Geometry: final body of the model. Coordinates: model frame, mm. A direction names the side the tool comes from. Give positions to 0.01 mm unless a question says otherwise; leave off trailing zeros. Write each loop counter-clockwise with the first axis right and the second up, starting at its lowest first coordinate (ties: lowest second). Pieces come first, ordered by that corner, then holes. Notation, with made-up numbers: (79.5, -28.5) -> (111.5, -28.5) arc R16 ccw to (111.5, -22.5) -> close; hole circle Ø7 at (75.25, -4). An arc over 180 degrees is marked (long way). Answer as a JSON object with one key per item and string values.
from build123d import *

# Parameters (mm, degrees)
SKETCH1_W               = 100
SKETCH1_H               = 100
BOSS_EXTRUDE1_DEPTH     = 100
SKETCH2_R               = 20
CUT_EXTRUDE1_DEPTH      = 5
CUT_EXTRUDE2_START      = -5
SKETCH3_R               = 20
CUT_EXTRUDE2_DEPTH      = 5
CUT_EXTRUDE3_DEPTH      = 151
CUT_EXTRUDE5_DEPTH      = 151
CUT_EXTRUDE5_DEPTH_BACK = 151
CUT_EXTRUDE6_DEPTH      = 151
CUT_EXTRUDE6_DEPTH_BACK = 151
FILLET3_R               = 2.5
BOSS_EXTRUDE3_DEPTH     = 10
CUT_EXTRUDE8_DEPTH      = 10
CUT_EXTRUDE9_DEPTH      = 10
BOSS_EXTRUDE4_DEPTH     = 10
CUT_EXTRUDE11_DEPTH     = 10
CUT_EXTRUDE12_DEPTH     = 10
BOSS_EXTRUDE5_DEPTH     = 10
CUT_EXTRUDE13_DEPTH     = 10
CUT_EXTRUDE15_DEPTH     = 10
BOSS_EXTRUDE6_DEPTH     = 10
CUT_EXTRUDE16_DEPTH     = 10
CUT_EXTRUDE17_DEPTH     = 10
BOSS_EXTRUDE7_DEPTH     = 10
CUT_EXTRUDE18_DEPTH     = 10
CUT_EXTRUDE19_DEPTH     = 10
BOSS_EXTRUDE8_DEPTH     = 10
CUT_EXTRUDE20_DEPTH     = 10
CUT_EXTRUDE21_DEPTH     = 10
BOSS_EXTRUDE9_DEPTH     = 10
CUT_EXTRUDE22_DEPTH     = 10
CUT_EXTRUDE23_DEPTH     = 10
BOSS_EXTRUDE10_DEPTH    = 10
CUT_EXTRUDE24_DEPTH     = 10
CUT_EXTRUDE25_DEPTH     = 10


with BuildPart() as part:
    # Sketch1 → Boss-Extrude1 (new body)
    with BuildSketch(Plane(origin=(0, 0, 0), x_dir=(0, 0, -1), z_dir=(1, 0, 0))):
        Rectangle(SKETCH1_W, SKETCH1_H)
    extrude(amount=BOSS_EXTRUDE1_DEPTH)

    # Sketch2 → Cut-Extrude1 (cut)
    with BuildSketch(Plane.ZY):
        Circle(SKETCH2_R)
    extrude(amount=-CUT_EXTRUDE1_DEPTH, mode=Mode.SUBTRACT)

    # Sketch3 → Cut-Extrude2 (cut)
    with BuildSketch(Plane(origin=(100, 0, 0), x_dir=(0, 0, -1), z_dir=(1, 0, 0)).offset(CUT_EXTRUDE2_START)):
        with Locations(Location((0, 0, 0), (0, 0, 180))):
            Circle(SKETCH3_R)
    extrude(amount=CUT_EXTRUDE2_DEPTH, mode=Mode.SUBTRACT)

    # Sketch4 → Cut-Extrude3 (cut, through all)
    with BuildSketch(Plane(origin=(0, 0, -50), x_dir=(-1, 0, 0), z_dir=(0, 0, -1))):
        Polygon((-80.128941466, 34.659382406), (-18.986632905, 34.659382406), (-9.691227462, 0), (-18.986632905, -35.340617594), (-80.128941466, -35.340617594), (-89.691227462, 0), align=None)
    extrude(amount=-CUT_EXTRUDE3_DEPTH, mode=Mode.SUBTRACT)

    # Sketch15 → Cut-Extrude5 (cut, two sides: drawn at the far end of the back side and taken through both)
    with BuildSketch(Plane(origin=(0, 50, 0), x_dir=(1, 0, 0), z_dir=(0, 1, 0)).offset(-CUT_EXTRUDE5_DEPTH_BACK)):
        with BuildLine():
            Line((75, -310), (75, -50))
            ThreePointArc((75, -50), (50, -25), (25, -50))
            Line((25, -50), (25, -310))
            Line((25, -310), (25, -830))
            Line((25, -830), (75, -830))
            Line((75, -830), (75, -310))
        make_face()
    extrude(amount=CUT_EXTRUDE5_DEPTH + CUT_EXTRUDE5_DEPTH_BACK, mode=Mode.SUBTRACT)

    # Sketch16 → Cut-Extrude6 (cut, two sides: drawn at the far end of the back side and taken through both)
    with BuildSketch(Plane(origin=(0, 50, 0), x_dir=(1, 0, 0), z_dir=(0, 1, 0)).offset(-CUT_EXTRUDE6_DEPTH_BACK)):
        with BuildLine():
            Line((25, 310), (25, 50))
            ThreePointArc((25, 50), (50, 25), (75, 50))
            Line((75, 50), (75, 310))
            Line((75, 310), (75, 830))
            Line((75, 830), (25, 830))
            Line((25, 830), (25, 310))
        make_face()
    extrude(amount=CUT_EXTRUDE6_DEPTH + CUT_EXTRUDE6_DEPTH_BACK, mode=Mode.SUBTRACT)

    # Fillet3
    fillet3_edges = [part.edges().sort_by_distance(p)[0] for p in [
        (50, -50, 25),
        (50, 50, 25),
        (50, -50, -25),
        (50, 50, -25),
    ]]
    fillet(fillet3_edges, radius=FILLET3_R)

    # Sketch17 → Boss-Extrude3 (add)
    with BuildSketch(Plane.XY.offset(50)):
        with BuildLine():
            Line((84.621199284, 43.079691203), (92.621199284, 43.079691203))
            ThreePointArc((92.621199284, 43.079691203), (94.621199284, 41.079691203), (92.621199284, 39.079691203))
            Line((92.621199284, 39.079691203), (84.621199284, 39.079691203))
            ThreePointArc((84.621199284, 39.079691203), (82.621199284, 41.079691203), (84.621199284, 43.079691203))
        make_face()
    extrude(amount=BOSS_EXTRUDE3_DEPTH)

    # Sketch18 → Cut-Extrude8 (cut)
    with BuildSketch(Plane(origin=(0, 43.079691203, 0), x_dir=(1, 0, 0), z_dir=(0, 1, 0))):
        Polygon((84.621199284, -50), (86.121199284, -60), (82.621199284, -60), (82.621199284, -50), align=None)
    extrude(amount=-CUT_EXTRUDE8_DEPTH, mode=Mode.SUBTRACT)

    # Sketch20 → Cut-Extrude9 (cut)
    with BuildSketch(Plane(origin=(0, 43.079691203, 0), x_dir=(1, 0, 0), z_dir=(0, 1, 0))):
        Polygon((91.121199284, -60), (94.621199284, -60), (94.621199284, -50), (92.621199284, -50), align=None)
    extrude(amount=-CUT_EXTRUDE9_DEPTH, mode=Mode.SUBTRACT)

    # Sketch24 → Boss-Extrude4 (add)
    with BuildSketch(Plane.XY.offset(50)):
        with BuildLine():
            Line((5.882221412, 43.579691203), (13.882221412, 43.579691203))
            ThreePointArc((13.882221412, 43.579691203), (16.382221412, 41.079691203), (13.882221412, 38.579691203))
            Line((13.882221412, 38.579691203), (5.882221412, 38.579691203))
            ThreePointArc((5.882221412, 38.579691203), (3.382221412, 41.079691203), (5.882221412, 43.579691203))
        make_face()
    extrude(amount=BOSS_EXTRUDE4_DEPTH)

    # Sketch25 → Cut-Extrude11 (cut)
    with BuildSketch(Plane(origin=(0, 43.579691203, 0), x_dir=(1, 0, 0), z_dir=(0, 1, 0))):
        Polygon((3.382221412, -50), (5.882221412, -50), (7.382221412, -60), (3.382221412, -60), align=None)
    extrude(amount=-CUT_EXTRUDE11_DEPTH, mode=Mode.SUBTRACT)

    # Sketch26 → Cut-Extrude12 (cut)
    with BuildSketch(Plane(origin=(0, 43.579691203, 0), x_dir=(1, 0, 0), z_dir=(0, 1, 0))):
        Polygon((12.382221412, -60), (13.882221412, -50), (16.382221412, -50), (16.382221412, -60), align=None)
    extrude(amount=-CUT_EXTRUDE12_DEPTH, mode=Mode.SUBTRACT)

    # Sketch27 → Boss-Extrude5 (add)
    with BuildSketch(Plane.XY.offset(50)):
        with BuildLine():
            Line((6.7978639, -43.920308797), (14.7978639, -43.920308797))
            ThreePointArc((14.7978639, -43.920308797), (17.2978639, -41.420308797), (14.7978639, -38.920308797))
            Line((14.7978639, -38.920308797), (6.7978639, -38.920308797))
            ThreePointArc((6.7978639, -38.920308797), (4.2978639, -41.420308797), (6.7978639, -43.920308797))
        make_face()
    extrude(amount=BOSS_EXTRUDE5_DEPTH)

    # Sketch29 → Cut-Extrude13 (cut)
    with BuildSketch(Plane.XZ.offset(43.920308797)):
        Polygon((8.2978639, 60), (6.7978639, 50), (4.2978639, 50), (4.2978639, 60), align=None)
    extrude(amount=-CUT_EXTRUDE13_DEPTH, mode=Mode.SUBTRACT)

    # Sketch30 → Cut-Extrude15 (cut)
    with BuildSketch(Plane.XZ.offset(43.920308797)):
        Polygon((14.0478639, 60), (17.2978639, 60), (17.2978639, 50), (14.7978639, 50), align=None)
    extrude(amount=-CUT_EXTRUDE15_DEPTH, mode=Mode.SUBTRACT)

    # Sketch31 → Boss-Extrude6 (add)
    with BuildSketch(Plane.XY.offset(50)):
        with BuildLine():
            Line((82.517325635, -38.920308797), (90.517325635, -38.920308797))
            ThreePointArc((90.517325635, -38.920308797), (93.017325635, -41.420308797), (90.517325635, -43.920308797))
            Line((90.517325635, -43.920308797), (82.517325635, -43.920308797))
            ThreePointArc((82.517325635, -43.920308797), (80.017325635, -41.420308797), (82.517325635, -38.920308797))
        make_face()
    extrude(amount=BOSS_EXTRUDE6_DEPTH)

    # Sketch33 → Cut-Extrude16 (cut)
    with BuildSketch(Plane.XZ.offset(43.920308797)):
        Polygon((83.621199284, 60), (82.517325635, 50), (80.017325635, 50), (80.017325635, 60), align=None)
    extrude(amount=-CUT_EXTRUDE16_DEPTH, mode=Mode.SUBTRACT)

    # Sketch34 → Cut-Extrude17 (cut)
    with BuildSketch(Plane.XZ.offset(43.920308797)):
        Polygon((89.56926246, 60), (90.517325635, 50), (93.017325635, 50), (93.017325635, 60), align=None)
    extrude(amount=-CUT_EXTRUDE17_DEPTH, mode=Mode.SUBTRACT)

    # Sketch35 → Boss-Extrude7 (add)
    with BuildSketch(Plane(origin=(0, 0, -50), x_dir=(-1, 0, 0), z_dir=(0, 0, -1))):
        with BuildLine():
            Line((-17.608468635, 43.579691203), (-9.608468635, 43.579691203))
            ThreePointArc((-9.608468635, 43.579691203), (-7.108468635, 41.079691203), (-9.608468635, 38.579691203))
            Line((-9.608468635, 38.579691203), (-17.608468635, 38.579691203))
            ThreePointArc((-17.608468635, 38.579691203), (-20.108468635, 41.079691203), (-17.608468635, 43.579691203))
        make_face()
    extrude(amount=BOSS_EXTRUDE7_DEPTH)

    # Sketch36 → Cut-Extrude18 (cut)
    with BuildSketch(Plane(origin=(0, 43.579691203, 0), x_dir=(1, 0, 0), z_dir=(0, 1, 0))):
        Polygon((11.108468635, 60), (9.608468635, 50), (7.108468635, 50), (7.108468635, 60), align=None)
    extrude(amount=-CUT_EXTRUDE18_DEPTH, mode=Mode.SUBTRACT)

    # Sketch37 → Cut-Extrude19 (cut)
    with BuildSketch(Plane(origin=(0, 43.579691203, 0), x_dir=(1, 0, 0), z_dir=(0, 1, 0))):
        Polygon((16.858468635, 60), (17.608468635, 50), (20.108468635, 50), (20.108468635, 60), align=None)
    extrude(amount=-CUT_EXTRUDE19_DEPTH, mode=Mode.SUBTRACT)

    # Sketch38 → Boss-Extrude8 (add)
    with BuildSketch(Plane(origin=(0, 0, -50), x_dir=(-1, 0, 0), z_dir=(0, 0, -1))):
        with BuildLine():
            Line((-17.330505729, -38.920308797), (-9.330505729, -38.920308797))
            ThreePointArc((-9.330505729, -38.920308797), (-6.830505729, -41.420308797), (-9.330505729, -43.920308797))
            Line((-9.330505729, -43.920308797), (-17.330505729, -43.920308797))
            ThreePointArc((-17.330505729, -43.920308797), (-19.830505729, -41.420308797), (-17.330505729, -38.920308797))
        make_face()
    extrude(amount=BOSS_EXTRUDE8_DEPTH)

    # Sketch40 → Cut-Extrude20 (cut)
    with BuildSketch(Plane.XZ.offset(43.920308797)):
        Polygon((10.830505729, -60), (9.330505729, -50), (6.830505729, -50), (6.830505729, -60), align=None)
    extrude(amount=-CUT_EXTRUDE20_DEPTH, mode=Mode.SUBTRACT)

    # Sketch41 → Cut-Extrude21 (cut)
    with BuildSketch(Plane.XZ.offset(43.920308797)):
        Polygon((16.580505729, -60), (17.330505729, -50), (19.830505729, -50), (19.830505729, -60), align=None)
    extrude(amount=-CUT_EXTRUDE21_DEPTH, mode=Mode.SUBTRACT)

    # Sketch42 → Boss-Extrude9 (add)
    with BuildSketch(Plane(origin=(0, 0, -50), x_dir=(-1, 0, 0), z_dir=(0, 0, -1))):
        with BuildLine():
            Line((-94.397005035, 43.579691203), (-86.397005035, 43.579691203))
            ThreePointArc((-86.397005035, 43.579691203), (-83.897005035, 41.079691203), (-86.397005035, 38.579691203))
            Line((-86.397005035, 38.579691203), (-94.397005035, 38.579691203))
            ThreePointArc((-94.397005035, 38.579691203), (-96.897005035, 41.079691203), (-94.397005035, 43.579691203))
        make_face()
    extrude(amount=BOSS_EXTRUDE9_DEPTH)

    # Sketch43 → Cut-Extrude22 (cut)
    with BuildSketch(Plane(origin=(0, 43.579691203, 0), x_dir=(1, 0, 0), z_dir=(0, 1, 0))):
        Polygon((87.897005035, 60), (86.397005035, 50), (83.897005035, 50), (83.897005035, 60), align=None)
    extrude(amount=-CUT_EXTRUDE22_DEPTH, mode=Mode.SUBTRACT)

    # Sketch44 → Cut-Extrude23 (cut)
    with BuildSketch(Plane(origin=(0, 43.579691203, 0), x_dir=(1, 0, 0), z_dir=(0, 1, 0))):
        Polygon((93.647005035, 60), (94.397005035, 50), (96.897005035, 50), (96.897005035, 60), align=None)
    extrude(amount=-CUT_EXTRUDE23_DEPTH, mode=Mode.SUBTRACT)

    # Sketch45 → Boss-Extrude10 (add)
    with BuildSketch(Plane(origin=(0, 0, -50), x_dir=(-1, 0, 0), z_dir=(0, 0, -1))):
        with BuildLine():
            Line((-93.140486024, -38.920308797), (-85.140486024, -38.920308797))
            ThreePointArc((-85.140486024, -38.920308797), (-82.640486024, -41.420308797), (-85.140486024, -43.920308797))
            Line((-85.140486024, -43.920308797), (-93.140486024, -43.920308797))
            ThreePointArc((-93.140486024, -43.920308797), (-95.640486024, -41.420308797), (-93.140486024, -38.920308797))
        make_face()
    extrude(amount=BOSS_EXTRUDE10_DEPTH)

    # Sketch47 → Cut-Extrude24 (cut)
    with BuildSketch(Plane.XZ.offset(43.920308797)):
        Polygon((86.640486024, -60), (85.140486024, -50), (82.640486024, -50), (82.640486024, -60), align=None)
    extrude(amount=-CUT_EXTRUDE24_DEPTH, mode=Mode.SUBTRACT)

    # Sketch48 → Cut-Extrude25 (cut)
    with BuildSketch(Plane.XZ.offset(43.920308797)):
        Polygon((91.647943496, -60), (93.140486024, -50), (95.640486024, -50), (95.640486024, -60), align=None)
    extrude(amount=-CUT_EXTRUDE25_DEPTH, mode=Mode.SUBTRACT)


solid = part.part
Q1. Material intervals for L1, parallel to Y at x = 1.7, z = 0; L2, parallel to Y at x = 46, z = -17; L3, parallel to X at y = -14, z = 36, sorted ascending. Write a range as from..to.
Values:
{"L1": "-50..-20, 20..50", "L2": "-50..-35.34, 34.66..50", "L3": "0..13.37, 85.9..100"}
Q2. Cut plane A-A (x = 50). Return the cut outline in (y, z), and give its area (3 significant figures).
Values:
{"outline": "(-50, -22.5) arc R2.5 ccw to (-47.5, -25) -> (-35.34, -25) -> (-35.34, 25) -> (-47.5, 25) arc R2.5 ccw to (-50, 22.5) -> close; (34.66, -25) -> (47.5, -25) arc R2.5 ccw to (50, -22.5) -> (50, 22.5) arc R2.5 ccw to (47.5, 25) -> (34.66, 25) -> close", "area": "1,490 mm²"}
Q3. Cut plane C-C (y = 2). Return the cut outline in (x, z).
Values:
{"outline": "(0, -50) -> (10.23, -50) -> (10.23, 50) -> (0, 50) -> (0, 19.9) -> (5, 19.9) -> (5, -19.9) -> (0, -19.9) -> close; (89.14, -50) -> (100, -50) -> (100, -19.9) -> (95, -19.9) -> (95, 19.9) -> (100, 19.9) -> (100, 50) -> (89.14, 50) -> close"}
Q4. Set-up query: faces 1 (the flat face through (7.56, -41.46, 55.07)), 2 (the flat face through (89, 43.08, 55)), 3 (the flat face through (14.274, -17.423, -0.7)), 4 (the flat face through (90, 43.58, -55)). Return all of +Z, -Z, +X, -X, +Y, -Y with unobstructed straight access to the full face (end or side cutting, diameter ignored); none if empty.
Values:
{"face 1": "+Z, -X, -Y", "face 2": "+Z, +X, +Y", "face 3": "+Z, -Z", "face 4": "-Z, +X, -X, +Y"}
Q5. First-contact query: P1, Ø3, axis at y = -4, z = 27, coming from the -X side; P2, Ø2.5, axis at x = 84.5, z = 53, coming from the -Y side; P3, Ø6.5, axis at x = 90, z = -54.5, coming from the +Y side; P4, Ø20, axis at y = -6, z = -5, coming from the +X side. Flat tips, straight axial feed; report the tip coordinate or a pass-through.
Values:
{"P1": "x = 0", "P2": "y = -43.92", "P3": "y = 43.58", "P4": "x = 95"}
Q6. Cut plane D-D (z = -52). Return the cut outline in (x, y).
Values:
{"outline": "(9.63, -43.92) -> (17.18, -43.92) -> (17.18, -38.92) -> (9.63, -38.92) -> close; (9.91, 38.58) -> (17.46, 38.58) -> (17.46, 43.58) -> (9.91, 43.58) -> close; (85.44, -43.92) -> (92.84, -43.92) -> (92.84, -38.92) -> (85.44, -38.92) -> close; (86.7, 38.58) -> (94.25, 38.58) -> (94.25, 43.58) -> (86.7, 43.58) -> close"}
Q7. Cut plane B-B (z = 0). Return the cut outline in (x, y), and give its area (3 significant figures).
Values:
{"outline": "(0, -50) -> (100, -50) -> (100, -20) -> (95, -20) -> (95, 20) -> (100, 20) -> (100, 50) -> (0, 50) -> (0, 20) -> (5, 20) -> (5, -20) -> (0, -20) -> close; hole (9.69, 0) -> (18.99, -35.34) -> (80.13, -35.34) -> (89.69, 0) -> (80.13, 34.66) -> (18.99, 34.66) -> close", "area": "4,660 mm²"}
Q8. Mould query, pull axis X, two halves, no side actions, for faces 5 (the flat face through (100, 23, 1)), 6 (the flat face through (6.62, 41.11, 54.93)), 7 (the flat face through (91, 41, -60)), 8 (the cylindrical face through (50.55, -41.505, 25.006)). Classes: pulls with the +X half, pulls with the -X half, needs draft (parallel to the pull), parting line crosses it, or undercut.
Values:
{"face 5": "pulls with the +X half", "face 6": "pulls with the -X half", "face 7": "needs draft", "face 8": "undercut"}
